from build123d import *

# Parameters (mm, degrees)
F1_DEPTH    = 30
F3_DEPTH    = 5
F4_T1_DEPTH = 34.125
F4_T4_ANGLE = 180
F4_T6_ANGLE = 180


# Not quite as in the source:
# - a fillet or chamfer that OpenCascade refuses, or shapes differently, is made with other operations: its cross-section is extruded or revolved along the edge and cut away or added


with BuildPart() as f1:
    # F0 (on Top) → F1 (new body)
    with BuildSketch(Plane.XY):
        with BuildLine():
            Line((-17.0625, -7.9375), (0, -7.9375))
            Line((0, -7.9375), (17.0625, -7.9375))
            ThreePointArc((17.0625, -7.9375), (25, 0), (17.0625, 7.9375))
            Line((17.0625, 7.9375), (0, 7.9375))
            Line((0, 7.9375), (-17.0625, 7.9375))
            ThreePointArc((-17.0625, 7.9375), (-25, 0), (-17.0625, -7.9375))
        make_face()
        with BuildLine():
            Line((-17.0625, 5.9375000447), (0, 5.9375000447))
            Line((0, 5.9375000447), (17.0625, 5.9375000447))
            ThreePointArc((17.0625, 5.9375000447), (23.0000000447, 0), (17.0625, -5.9375000447))
            Line((17.0625, -5.9375000447), (0, -5.9375000447))
            Line((0, -5.9375000447), (-17.0625, -5.9375000447))
            ThreePointArc((-17.0625, -5.9375000447), (-23.0000000447, 0), (-17.0625, 5.9375000447))
        make_face(mode=Mode.SUBTRACT)
    extrude(amount=F1_DEPTH)

    # F2 (on face) → F3 (join)
    with BuildSketch(Plane.XY.offset(30)):
        with BuildLine():
            ThreePointArc((17.0625, -10.9375000447), (28.0000000447, 0), (17.0625, 10.9375000447))
            Line((17.0625, 10.9375000447), (-17.0625, 10.9375000447))
            ThreePointArc((-17.0625, 10.9375000447), (-28.0000000447, 0), (-17.0625, -10.9375000447))
            Line((-17.0625, -10.9375000447), (17.0625, -10.9375000447))
        make_face()
        with BuildLine():
            Line((17.0625, -7.9375), (-17.0625, -7.9375))
            ThreePointArc((-17.0625, -7.9375), (-25, 0), (-17.0625, 7.9375))
            Line((-17.0625, 7.9375), (17.0625, 7.9375))
            ThreePointArc((17.0625, 7.9375), (25, 0), (17.0625, -7.9375))
        make_face(mode=Mode.SUBTRACT)
        with BuildLine():
            ThreePointArc((-17.0625, 7.9375), (-25, 0), (-17.0625, -7.9375))
            Line((-17.0625, -7.9375), (17.0625, -7.9375))
            ThreePointArc((17.0625, -7.9375), (25, 0), (17.0625, 7.9375))
            Line((17.0625, 7.9375), (-17.0625, 7.9375))
        make_face()
        with BuildLine():
            Line((-17.0625, 5.9375000447), (17.0625, 5.9375000447))
            ThreePointArc((17.0625, 5.9375000447), (23.0000000447, 0), (17.0625, -5.9375000447))
            Line((17.0625, -5.9375000447), (-17.0625, -5.9375000447))
            ThreePointArc((-17.0625, -5.9375000447), (-23.0000000447, 0), (-17.0625, 5.9375000447))
        make_face(mode=Mode.SUBTRACT)
    extrude(amount=F3_DEPTH)

    # F4: chamfer of 4 x 2.3094010768 on 4 edges, made by hand

    # F4_s2 → F4_t1 (cut)
    with BuildSketch(Plane.YZ.offset(-17.0625)):
        Polygon((-8.6280989679, 35), (-10.9375000447, 31), (-10.9375000447, 35), align=None)
        Polygon((8.6280989679, 35), (10.9375000447, 31), (10.9375000447, 35), align=None)
    extrude(amount=F4_T1_DEPTH, mode=Mode.SUBTRACT)

    # F4_s3 → F4_t4 (revolve, cut)
    with BuildSketch(Plane.YZ.offset(-17.0625)):
        Polygon((8.6280989679, 35), (10.9375000447, 31), (10.9375000447, 35), align=None)
    revolve(axis=Axis((-17.0625, 0, 35), (0, 0, 1)), revolution_arc=F4_T4_ANGLE, mode=Mode.SUBTRACT)

    # F4_s5 → F4_t6 (revolve, cut)
    with BuildSketch(Plane.YZ.offset(17.0625)):
        Polygon((-8.6280989679, 35), (-10.9375000447, 31), (-10.9375000447, 35), align=None)
    revolve(axis=Axis((17.0625, 0, 35), (0, 0, 1)), revolution_arc=F4_T6_ANGLE, mode=Mode.SUBTRACT)


solid = f1.part
The listing builds one solid part. Answer for the finished solid, in the listing's coordinates (mm). A direction names the side the tool comes from. Round coordinates to 2 decimals unless told otherwise and drop trailing zeros. Write each loop counter-clockwise with the first axis right and the second up, starting at its lowest first coordinate (ties: lowest second). Pieces come first, ordered by that corner, then holes. Notation, with made-up numbers: (23.25, 38.25) - (67.25, 38.25) arc R23 ccw to (67.25, 74.25) - close; hole circle Ø10 at (-14, -18). An arc over 180 degrees is marked (long way). Use a Markdown table: item, result. Add a question column.
1. A tool of negligible diameter and unlimited length cuts with its end or side. For faces 5 (the face through (25, 0, 15)), 6 (the face through (-0.1, -8.1, 30)), 7 (the face through (0, 5.938, 17)), from which of +Z, -Z, +X, -X, +Y, -Y can it reach the whole face along a straight path? Write none if from no direction.
2. The part is cut by section C-C (x = 13). Write down the section's boundary in (y, z).
3. The part is cut by section B-B (y = 0). Write down the section's boundary in (x, z), and give its area (3 significant figures).
4. Flat-ended cylindrical pins translate along their axes: P1, Ø10, axis at x = 0, z = 21.5, coming from the -Y side; P2, Ø2, axis at y = -7.5, z = 25, coming from the -X side; P3, Ø2, axis at y = 5.5, z = 15.5, coming from the -X side. Find the tip coordinate at first contact, or state that the pin passes through.
5. For a pull along Y with two mould halves and no side action, classify faces 1 (the face through (-23, 0, 17)), 2 (the face through (0, -5.938, 17)), 3 (the face through (28, -0.2, 30.5)), 4 (the face through (0, 7, 0)) as +Y half, -Y half, draft (parallel to the pull), parting line (faces both ways), or undercut.
6. The part is cut by section A-A (z = 18). Write down the section's boundary in (x, y) (1 decimal), and give its area (3 significant figures).
7. Consider line 1 (Y direction, x = -2, z = 6.5); line 2 (X direction, y = 0.5, z = 10.5); line 3 (Y direction, x = 19.5, z = 26). Determine where each line is inside the solid, lowest interval first.
Reported:
| question | item | result |
|---|---|---|
| 1 | face 5 | -Z, +X |
| 1 | face 6 | -Z |
| 1 | face 7 | +Z, -Z |
| 2 | outline | (-10.94, 30) - (-7.94, 30) - (-7.94, 0) - (-5.94, 0) - (-5.94, 35) - (-8.63, 35) - (-10.94, 31) - close; (5.94, 0) - (7.94, 0) - (7.94, 30) - (10.94, 30) - (10.94, 31) - (8.63, 35) - (5.94, 35) - close |
| 3 | outline | (-28, 30) - (-25, 30) - (-25, 0) - (-23, 0) - (-23, 35) - (-25.69, 35) - (-28, 31) - close; (23, 0) - (25, 0) - (25, 30) - (28, 30) - (28, 31) - (25.69, 35) - (23, 35) - close |
| 3 | area | 161 mm^2 |
| 4 | P1 | y = -7.94 |
| 4 | P2 | x = -21.62 |
| 4 | P3 | x = -23.6 |
| 5 | face 1 | undercut |
| 5 | face 2 | undercut |
| 5 | face 3 | parting line |
| 5 | face 4 | draft |
| 6 | outline | (-17.1, -7.9) - (17.1, -7.9) arc R7.9 ccw to (17.1, 7.9) - (-17.1, 7.9) arc R7.9 ccw to start; hole (-17.1, -5.9) - (17.1, -5.9) arc R5.9 ccw to (17.1, 5.9) - (-17.1, 5.9) arc R5.9 ccw to start |
| 6 | area | 224 mm^2 |
| 7 | line 1 | -7.94 to -5.94, 5.94 to 7.94 |
| 7 | line 2 | -24.98 to -22.98, 22.98 to 24.98 |
| 7 | line 3 | -7.55 to -5.41, 5.41 to 7.55 |
